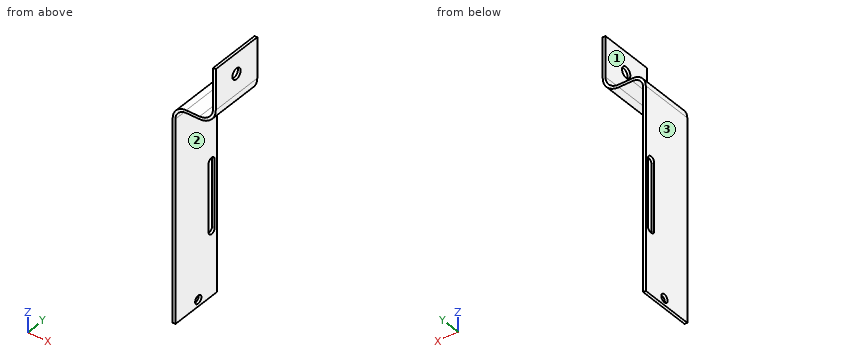
from build123d import *

# Parameters (mm, degrees)
EXTRUDE_THIN1_DEPTH = 20
SKETCH2_R           = 2
CUT_EXTRUDE1_DEPTH  = 17
SKETCH3_R           = 1.5
CUT_EXTRUDE2_DEPTH  = 2
CUT_EXTRUDE3_DEPTH  = 17


with BuildPart() as part:
    # Sketch1 → Extrude-Thin1 (new body)
    with BuildSketch(Plane(origin=(0, 0, 0), x_dir=(1, 0, 0), z_dir=(0, 1, 0))):
        with BuildLine():
            Line((0, 0), (0, 15))
            ThreePointArc((0, 15), (-1.464466094, 18.535533906), (-5, 20))
            Line((-5, 20), (-10, 20))
            ThreePointArc((-10, 20), (-13.535533906, 21.464466094), (-15, 25))
            Line((-15, 25), (-15, 100))
            Line((-15, 100), (-14, 100))
            Line((-14, 100), (-14, 25))
            ThreePointArc((-14, 25), (-12.828427125, 22.171572875), (-10, 21))
            Line((-10, 21), (-5, 21))
            ThreePointArc((-5, 21), (-0.757359313, 19.242640687), (1, 15))
            Line((1, 15), (1, 0))
            Line((1, 0), (0, 0))
        make_face()
    extrude(amount=EXTRUDE_THIN1_DEPTH)

    # Sketch2 → Cut-Extrude1 (cut, through all)
    with BuildSketch(Plane(origin=(1, 0, 0), x_dir=(0, 0, -1), z_dir=(1, 0, 0))):
        with Locations((7.5, 10)):
            Circle(SKETCH2_R)
    extrude(amount=-CUT_EXTRUDE1_DEPTH, mode=Mode.SUBTRACT)

    # Sketch3 → Cut-Extrude2 (cut, through all)
    with BuildSketch(Plane(origin=(-14, 0, 0), x_dir=(0, 0, -1), z_dir=(1, 0, 0))):
        with Locations((97.5, 11)):
            Circle(SKETCH3_R)
    extrude(amount=-CUT_EXTRUDE2_DEPTH, mode=Mode.SUBTRACT)

    # Sketch4 → Cut-Extrude3 (cut, through all)
    with BuildSketch(Plane.ZY.offset(15)):
        with BuildLine():
            Line((-50.783321534, 18.959123293), (-75.783321534, 18.959123293))
            ThreePointArc((-75.783321534, 18.959123293), (-77.283321534, 17.459123293), (-75.783321534, 15.959123293))
            Line((-75.783321534, 15.959123293), (-50.783321534, 15.959123293))
            ThreePointArc((-50.783321534, 15.959123293), (-49.283321534, 17.459123293), (-50.783321534, 18.959123293))
        make_face()
    extrude(amount=-CUT_EXTRUDE3_DEPTH, mode=Mode.SUBTRACT)


solid = part.part
The listing builds one solid part. Answer for the finished solid, in the listing's coordinates (mm). Face numbers are marked on the shaded views. A direction names the side the tool comes from. Coordinates: 2 decimals unless noted, no trailing zeros. Loops run counter-clockwise (first coordinate to the right, second up) from the corner with the lowest first, then second, coordinate; pieces in that order, holes last. Notation, with made-up numbers: M 79,72 L 135,72 A34 cw 135,109 Z; hole C 45,-25 d9. An arc over 180 degrees is marked long. Answer in a Markdown table with one row per item.
1) Find section D-D (z = -97.5). Determine the outline of the cut face in (x, y).
Answers below:
| item | result |
|---|---|
| outline | M -15,0 L -14,0 L -14,9.5 L -15,9.5 Z; M -15,12.5 L -14,12.5 L -14,20 L -15,20 Z |
2) Which of the six approach directions +Z, -Z, +X, -X, +Y, -Y give full straight-line access (tool end or side, diameter ignored) to the marked faces 1, 2 and 3?
Answers below:
| item | result |
|---|---|
| face 1 | +Z, -X, +Y, -Y |
| face 2 | -Z, +X, +Y, -Y |
| face 3 | +Z, -Z, -X, +Y, -Y |
3) Find section C-C (y = 18). Determine the outline of the cut face in (x, z), then the cut area to 3 significant figures.
Answers below:
| item | result |
|---|---|
| outline | M -15,-100 L -14,-100 L -14,-77.18 L -15,-77.18 Z; M -15,-49.38 L -14,-49.38 L -14,-25 A4 cw -10,-21 L -5,-21 A6 ccw 1,-15 L 1,0 L 0,0 L 0,-15 A5 cw -5,-20 L -10,-20 A5 ccw -15,-25 Z |
| area | 82.9 mm^2 |
4) Find section A-A (z = -7.5). Determine the outline of the cut face in (x, y), then the cut area to 3 significant figures.
Answers below:
| item | result |
|---|---|
| outline | M 0,0 L 1,0 L 1,8 L 0,8 Z; M 0,12 L 1,12 L 1,20 L 0,20 Z |
| area | 16.0 mm^2 |
5) Find section B-B (y = 2.25). Determine the outline of the cut face in (x, z).
Answers below:
| item | result |
|---|---|
| outline | M -15,-100 L -14,-100 L -14,-25 A4 cw -10,-21 L -5,-21 A6 ccw 1,-15 L 1,0 L 0,0 L 0,-15 A5 cw -5,-20 L -10,-20 A5 ccw -15,-25 Z |
6) Find the intervals of material crossed by probe 1 along Y at (x, z) = (0.4, -7.5); probe 2 along X at (y, z) = (1.5, -8); probe 3 along X at (y, z) = (15, -41), in increasing order.
Answers below:
| item | result |
|---|---|
| probe 1 | 0 to 8, 12 to 20 |
| probe 2 | 0 to 1 |
| probe 3 | -15 to -14 |
7) Given pin 1 (4 mm diameter, centred on y = 4, z = -31, fed in from +X); pin 2 (2.5 mm diameter, centred on x = -7.5, y = 7, fed in from +Z); pin 3 (1.5 mm diameter, centred on x = -8.5, y = 5.5, fed in from -Z), each flat-ended and moving along its own axis, determine where each tip first touches the part or whether it passes through.
Answers below:
| item | result |
|---|---|
| pin 1 | x = -14 |
| pin 2 | z = -20 |
| pin 3 | z = -21 |
